Here's how the part is built. I have some questions about the finished solid (model axes, mm). A direction names the side the tool comes from. Coordinates: 2 decimals unless noted, no trailing zeros. Write each loop counter-clockwise with the first axis right and the second up, starting at its lowest first coordinate (ties: lowest second). Pieces come first, ordered by that corner, then holes. Notation, with made-up numbers: (58.5, 72.25) - (94.5, 72.25) arc R16 ccw to (94.5, 79.25) - close; hole circle Ø1 at (30.25, 28). An arc over 180 degrees is marked (long way). Answer in a Markdown table with one row per item. Add a question column.
Item 1: If I drill on probe 1 along Y at (x, z) = (13, -3.5); probe 2 along X at (y, z) = (2.45, -95.5); probe 3 along Y at (x, z) = (11.5, -36.5), over which ranges is the centre line in solid material (lowest first)? Write a range as from..to.
Item 2: We'd pull the mould along X, two halves only. Please class faces 1 (the face through (5, 2, -100.5)), 2 (the face through (26.25, 9.53, -2.46)), 3 (the face through (33.63, 2.54, -42.12)): +X half, -X half, draft (parallel to the pull), parting line (faces both ways), or undercut.
Item 3: Imagine slicing it at D-D (x = 23). Please give me the cut outline in (y, z).
Item 4: Which directions (+Z, -Z, +X, -X, +Y, -Y) give clear straight access to the entire face, cutting with the end or side of a thin tool? Please do faces 4 (the face through (21.5, 14, -38)), 5 (the face through (30, 24.45, -3)), 6 (the face through (12, 5, -53)).
Item 5: I'm going to push flat-ended pins straight in: pin 1 (3.5 mm diameter, centred on y = 27, z = -3, fed in from -X); pin 2 (8 mm diameter, centred on y = 5.5, z = -18, fed in from +X); pin 3 (3 mm diameter, centred on x = 13, y = 9.45, fed in from +Z); pin 4 (3.5 mm diameter, centred on x = 13, y = 22, fed in from -Z). Where does each tip first touch, or does it pass through?
Item 6: Imagine slicing it at C-C (z = -74.5). Please give me the cut outline in (x, y), plus the area to 3 significant figures.
Item 7: Imagine slicing it at A-A (x = 5). Please give me the cut outline in (y, z).
Item 8: Imagine slicing it at B-B (y = 19.45). Please give me the cut outline in (x, z).
from build123d import *

# Parameters (mm, degrees)
SKETCH1_W           = 41
SKETCH1_H           = 100.5
BOSS_EXTRUDE1_DEPTH = 5
SKETCH2_W           = 21
SKETCH2_H           = 10.2
CUT_EXTRUDE1_DEPTH  = 6
SKETCH9_R           = 1.75
CUT_EXTRUDE4_DEPTH  = 6
CUT_EXTRUDE5_DEPTH  = 6
BOSS_EXTRUDE4_DEPTH = 23.9
SKETCH16_W          = 2
SKETCH16_H          = 85.3
BOSS_EXTRUDE5_DEPTH = 23.9
CUT_EXTRUDE8_DEPTH  = 22.5
BOSS_EXTRUDE6_DEPTH = 28.9
SKETCH25_W          = 6.53486924
SKETCH25_H          = 4.45
CUT_EXTRUDE9_DEPTH  = 6
SKETCH26_R          = 1.75
CUT_EXTRUDE10_DEPTH = 101.5


with BuildPart() as part:
    # Sketch1 → Boss-Extrude1 (new body)
    with BuildSketch(Plane(origin=(0, 0, 0), x_dir=(1, 0, 0), z_dir=(0, 1, 0))):
        with Locations((20.5, 50.25)):
            Rectangle(SKETCH1_W, SKETCH1_H)
    extrude(amount=BOSS_EXTRUDE1_DEPTH)

    # Sketch2 → Cut-Extrude1 (cut, through all)
    with BuildSketch(Plane(origin=(0, 5, 0), x_dir=(1, 0, 0), z_dir=(0, 1, 0))):
        with Locations((20.5, 95.4)):
            Rectangle(SKETCH2_W, SKETCH2_H)
    extrude(amount=-CUT_EXTRUDE1_DEPTH, mode=Mode.SUBTRACT)

    # Sketch9 → Cut-Extrude4 (cut, through all)
    with BuildSketch(Plane(origin=(0, 5, 0), x_dir=(1, 0, 0), z_dir=(0, 1, 0))):
        with Locations((5, 95.5)):
            Circle(SKETCH9_R)
        with Locations((36, 95.5)):
            Circle(SKETCH9_R)
    extrude(amount=-CUT_EXTRUDE4_DEPTH, mode=Mode.SUBTRACT)

    # Sketch11 → Cut-Extrude5 (cut, through all)
    with BuildSketch(Plane(origin=(0, 5, 0), x_dir=(1, 0, 0), z_dir=(0, 1, 0))):
        Polygon((15.5, 0), (0, 80.3), (0, 0), align=None)
        Polygon((25.5, 0), (41, 80.3), (41, 0), align=None)
    extrude(amount=-CUT_EXTRUDE5_DEPTH, mode=Mode.SUBTRACT)

    # Sketch12 → Boss-Extrude4 (add)
    with BuildSketch(Plane(origin=(0, 5, 0), x_dir=(1, 0, 0), z_dir=(0, 1, 0))):
        Polygon((25.5, 0), (15.5, 0), (14.53486924, 5), (26.46513076, 5), align=None)
    extrude(amount=BOSS_EXTRUDE4_DEPTH)

    # Sketch16 → Boss-Extrude5 (add)
    with BuildSketch(Plane(origin=(0, 5, 0), x_dir=(1, 0, 0), z_dir=(0, 1, 0))):
        with Locations((20.5, 47.65)):
            Rectangle(SKETCH16_W, SKETCH16_H)
    extrude(amount=BOSS_EXTRUDE5_DEPTH)

    # Sketch17 → Cut-Extrude8 (cut, through all)
    with BuildSketch(Plane.ZY.offset(-19.5)):
        Polygon((-90.4, 5), (-5, 28.9), (-90.3, 28.9), align=None)
    extrude(amount=-CUT_EXTRUDE8_DEPTH, mode=Mode.SUBTRACT)

    # Sketch23 → Boss-Extrude6 (add)
    with BuildSketch(Plane(origin=(0, 28.9, 0), x_dir=(1, 0, 0), z_dir=(0, 1, 0))):
        Polygon((26.46513076, 5), (33, 5), (33, 0), (25.5, 0), align=None)
        Polygon((14.53486924, 5), (8, 5), (8, 0), (15.5, 0), align=None)
    extrude(amount=-BOSS_EXTRUDE6_DEPTH)

    # Sketch25 → Cut-Extrude9 (cut, through all)
    with BuildSketch(Plane(origin=(0, 0, -5), x_dir=(-1, 0, 0), z_dir=(0, 0, -1))):
        with Locations((-11.26743462, 2.225)):
            Rectangle(SKETCH25_W, SKETCH25_H)
        with Locations((-29.73256538, 2.225)):
            Rectangle(SKETCH25_W, SKETCH25_H)
        with Locations((-11.26743462, 26.675)):
            Rectangle(SKETCH25_W, SKETCH25_H)
        with Locations((-29.73256538, 26.675)):
            Rectangle(SKETCH25_W, SKETCH25_H)
    extrude(amount=-CUT_EXTRUDE9_DEPTH, mode=Mode.SUBTRACT)

    # Sketch26 → Cut-Extrude10 (cut, through all)
    with BuildSketch(Plane.XY):
        with Locations((13, 19.45)):
            Circle(SKETCH26_R)
        with Locations((28, 19.45)):
            Circle(SKETCH26_R)
        with Locations((13, 9.45)):
            Circle(SKETCH26_R)
        with Locations((28, 9.45)):
            Circle(SKETCH26_R)
    extrude(amount=-CUT_EXTRUDE10_DEPTH, mode=Mode.SUBTRACT)


solid = part.part
Here are the results:
| question | item | result |
|---|---|---|
| 1 | probe 1 | y = 4.45..7.7, 11.2..17.7, 21.2..24.45 |
| 1 | probe 2 | x = 0..3.25, 6.75..10, 31..34.25, 37.75..41 |
| 1 | probe 3 | y = 0..5 |
| 2 | face 1 | draft |
| 2 | face 2 | undercut |
| 2 | face 3 | +X half |
| 3 | outline | (0, -90.3) - (5, -90.3) - (5, -5) - (28.9, -5) - (28.9, 0) - (0, 0) - close |
| 4 | face 4 | -Z, +X, +Y |
| 4 | face 5 | +Z, -Z, +X, +Y |
| 4 | face 6 | -Z, -X, +Y |
| 5 | pin 1 | stops at x = 14.53 |
| 5 | pin 2 | stops at x = 29.74 |
| 5 | pin 3 | passes through |
| 5 | pin 4 | stops at z = -5 |
| 6 | outline | (1.12, 0) - (39.88, 0) - (39.88, 5) - (21.5, 5) - (21.5, 9.45) - (19.5, 9.45) - (19.5, 5) - (1.12, 5) - close |
| 6 | area | 203 mm2 |
| 7 | outline | (0, -100.5) - (5, -100.5) - (5, -97.25) - (0, -97.25) - close; (0, -93.75) - (5, -93.75) - (5, -54.4) - (0, -54.4) - close |
| 8 | outline | (8, -5) - (11.25, -5) - (11.25, 0) - (8, 0) - close; (14.75, -5) - (19.5, -5) - (19.5, -38.77) - (21.5, -38.77) - (21.5, -5) - (26.25, -5) - (26.25, 0) - (14.75, 0) - close; (29.75, -5) - (33, -5) - (33, 0) - (29.75, 0) - close |
